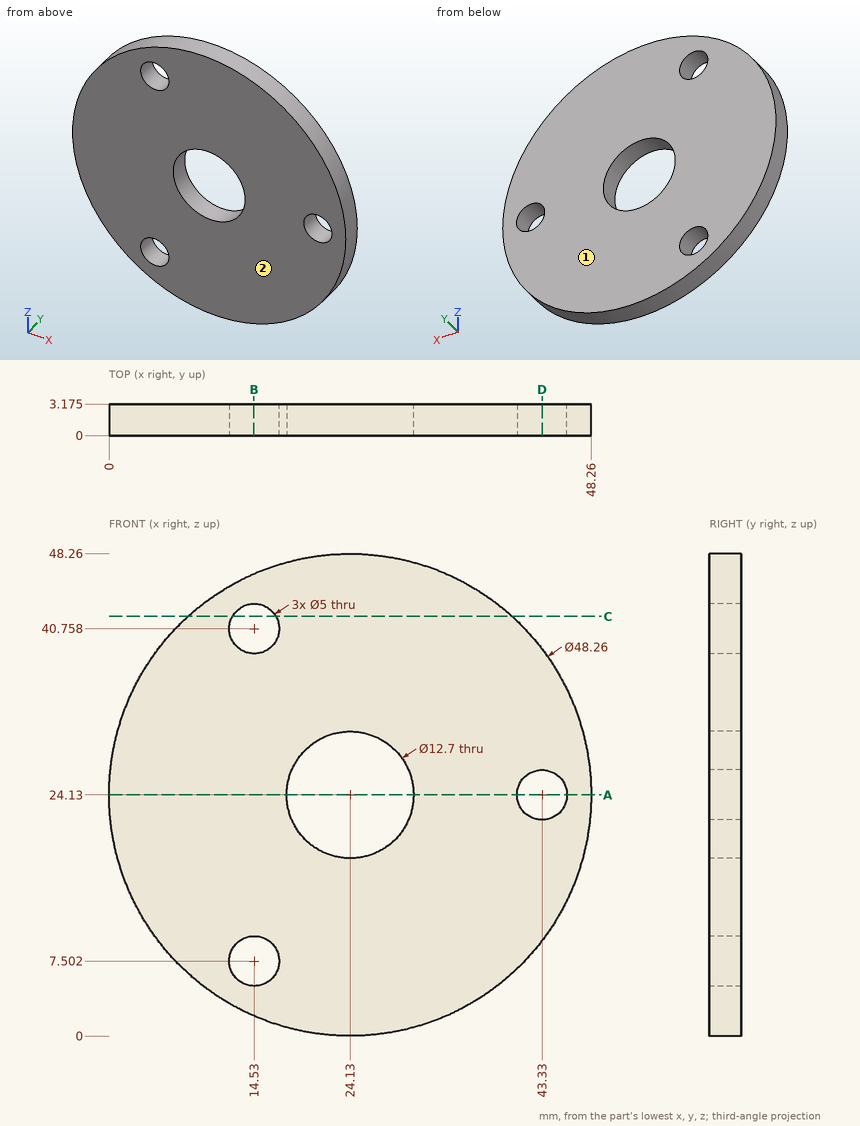
Could you check a few things on this drawing? It's one solid part, dimensions in mm from its lowest x, y, z. Round coordinates to 2 decimals unless told otherwise and drop trailing zeros. Loops run counter-clockwise (first coordinate to the right, second up) from the corner with the lowest first, then second, coordinate; pieces in that order, holes last.
Q1. For P1, Ø3, axis at x = 43.33, z = 24.13, coming from the +Y side; P2, Ø1.5, axis at y = 2.5, z = 14, coming from the -X side; P3, Ø1, axis at x = 5, y = 3, coming from the +Z side (1 decimal); P4, Ø1, axis at x = 29, y = 2, coming from the -Z side, each with a flat end and sliding along its axis, tell me the tip position at first contact or that it passes through.
Q2. I want a section at C-C (z = 42). Write out the boundary of the cut face in (x, y) (1 decimal).
Q3. I want a section at B-B (x = 14.5). Write out the boundary of the cut face in (y, z) (1 decimal), and give its area (3 significant figures).
Q4. I want a section at A-A (z = 24.13). Write out the boundary of the cut face in (x, y) (1 decimal).
Q5. I want a section at D-D (x = 43.33). Write out the boundary of the cut face in (y, z) (1 decimal).
Q6. Please list where these lines run through material, in increasing order: L1, parallel to X at y = 1.6, z = 24.13; L2, parallel to Z at x = 13.5, y = 0.95 (1 decimal); L3, parallel to Z at x = 24, y = 2.6.
Q7. Thinking about a two-plate mould opening in Y: for the marked faces 1 and 2, which applies, pulls with the +Y half, pulls with the -Y half, needs draft (parallel to the pull), parting line crosses it, or undercut?
Answer below:
1. P1: passes through
1. P2: stops at x = 1.9
1. P3: stops at z = 39.5
1. P4: stops at z = 0.4
2. outline: (7.9, 0) - (12.4, 0) - (12.4, 3.2) - (7.9, 3.2) - close; (16.7, 0) - (40.3, 0) - (40.3, 3.2) - (16.7, 3.2) - close
3. outline: (0, 2) - (3.2, 2) - (3.2, 5) - (0, 5) - close; (0, 10) - (3.2, 10) - (3.2, 38.3) - (0, 38.3) - close; (0, 43.3) - (3.2, 43.3) - (3.2, 46.3) - (0, 46.3) - close
3. area: 109 mm2
4. outline: (0, 0) - (17.8, 0) - (17.8, 3.2) - (0, 3.2) - close; (30.5, 0) - (40.8, 0) - (40.8, 3.2) - (30.5, 3.2) - close; (45.8, 0) - (48.3, 0) - (48.3, 3.2) - (45.8, 3.2) - close
5. outline: (0, 9.5) - (3.2, 9.5) - (3.2, 21.6) - (0, 21.6) - close; (0, 26.6) - (3.2, 26.6) - (3.2, 38.7) - (0, 38.7) - close
6. L1: x = 0 to 17.78, 30.48 to 40.83, 45.83 to 48.26
6. L2: z = 2.5 to 5.2, 9.8 to 38.5, 43 to 45.8
6. L3: z = 0 to 17.78, 30.48 to 48.26
7. face 1: pulls with the +Y half
7. face 2: pulls with the -Y half
